Can you work these out from the model? Positions are in its coordinate system, mm. Coordinates: 2 decimals unless noted, no trailing zeros. Write each loop counter-clockwise with the first axis right and the second up, starting at its lowest first coordinate (ties: lowest second). Pieces come first, ordered by that corner, then holes. Notation, with made-up numbers: M -19.5,68.5 L 10.5,68.5 A19 ccw 10.5,82.5 Z; hole C 72,-6 d4. An arc over 180 degrees is marked long. Use one line per item in the form item = value. Start each with the question number.
```python
from build123d import *

# Parameters (mm, degrees)
F0_W     = 6.408992
F0_H     = 7.585215
F1_DEPTH = 2.54


with BuildPart() as f1:
    # F0 (on Front) → F1 (new body)
    with BuildSketch(Plane.XZ):
        Polygon((-12.7, 0), (0, 0), (12.7, 0), (12.7, 93.983997), (10.482716, 93.983997), (-10.482716, 93.983997), (-12.7, 93.983997), align=None)
        Polygon((-10.482716, 109.624464), (-10.482716, 93.983997), (10.482716, 93.983997), (10.482716, 109.624464), (5.35761, 109.624464), (-5.35761, 109.624464), align=None)
        Polygon((-5.35761, 117.408185), (-5.35761, 109.624464), (5.35761, 109.624464), (5.35761, 117.408185), (3.204496, 117.408185), (-3.204496, 117.408185), align=None)
        with Locations((0, 121.200792)):
            Rectangle(F0_W, F0_H)
    extrude(amount=-F1_DEPTH)


solid = f1.part
```
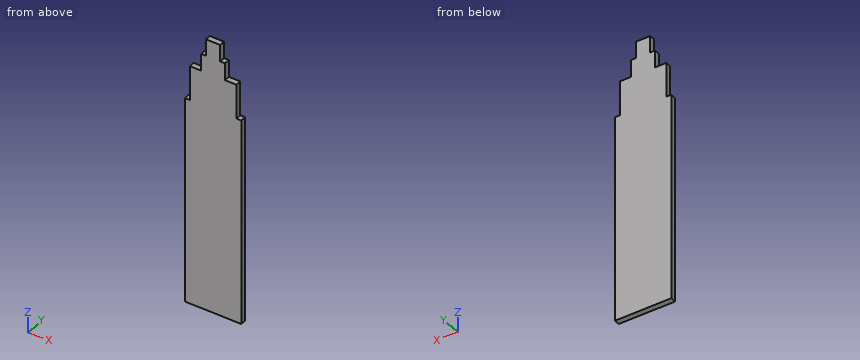
1) Suppose I cut it at C-C on z = 106. Please give me the cut outline in (x, y), and give its area (3 significant figures).
2) Suppose I cut it at B-B on x = -8.25. Please give me the cut outline in (y, z), and give its area (3 significant figures).
3) Suppose I cut it at A-A on y = 1.75. Please give me the cut outline in (x, z).
4) Please list where these lines run through material, in increasing order: line 1 (Z direction, x = 7.75, y = 1.15); line 2 (X direction, y = 1.7, z = 111); line 3 (X direction, y = 0.9, z = 108).
5) Will these pins go through, and if not, where does the flat tip stop? pin 1 Ø1.3 at (y, z) = (2, 123) entering from +X; pin 2 Ø1.1 at (x, y) = (-12, 1) entering from +Z; pin 3 Ø0.8 at (x, y) = (7.5, 1.5) entering from +Z.
Computed values:
q1.outline = M -10.48,0 L 10.48,0 L 10.48,2.54 L -10.48,2.54 Z
q1.area = 53.3 mm²
q2.outline = M 0,0 L 2.54,0 L 2.54,109.62 L 0,109.62 Z
q2.area = 278 mm²
q3.outline = M -12.7,0 L 12.7,0 L 12.7,93.98 L 10.48,93.98 L 10.48,109.62 L 5.36,109.62 L 5.36,117.41 L 3.2,117.41 L 3.2,124.99 L -3.2,124.99 L -3.2,117.41 L -5.36,117.41 L -5.36,109.62 L -10.48,109.62 L -10.48,93.98 L -12.7,93.98 Z
q4.line_1 = 0 to 109.62
q4.line_2 = -5.36 to 5.36
q4.line_3 = -10.48 to 10.48
q5.pin_1 = 3.2
q5.pin_2 = 93.98
q5.pin_3 = 109.62
